Geometry check sheet. Reference: the model listing, model coordinates, mm. Face numbers are marked on the shaded views. Coordinates: 2 decimals unless noted, no trailing zeros. Loops run counter-clockwise (first coordinate to the right, second up) from the corner with the lowest first, then second, coordinate; pieces in that order, holes last. Notation, with made-up numbers: (60, 72.25) -> (116, 72.25) arc R16 ccw to (116, 88.25) -> close; hole circle Ø7 at (-36, -5). An arc over 180 degrees is marked (long way). Answer as a JSON object with one key per item and string values.
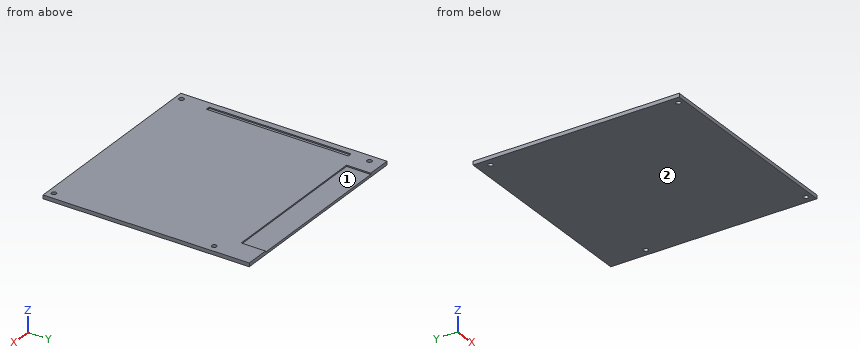
from build123d import *

# Parameters (mm, degrees)
F0_W     = 170
F0_H     = 170
F0_R     = 1.98
F1_DEPTH = 3
F2_W     = 130
F2_H     = 20
F3_DEPTH = 1
F4_W     = 3.516979
F4_H     = 117.000129
F5_DEPTH = 1


with BuildPart() as f1:
    # F0 (on Top) → F1 (new body)
    with BuildSketch(Plane.XY):
        Rectangle(F0_W, F0_H)
        with Locations((-78.65, -80.1)):
            Circle(F0_R, mode=Mode.SUBTRACT)
        with Locations((78.83, -80.1)):
            Circle(F0_R, mode=Mode.SUBTRACT)
        with Locations((-78.65, 74.84)):
            Circle(F0_R, mode=Mode.SUBTRACT)
        with Locations((78.83, 51.98)):
            Circle(F0_R, mode=Mode.SUBTRACT)
    extrude(amount=F1_DEPTH)

    # F2 (on face) → F3 (cut)
    with BuildSketch(Plane.XY.offset(3)):
        with Locations((0, 75)):
            Rectangle(F2_W, F2_H)
    extrude(amount=-F3_DEPTH, mode=Mode.SUBTRACT)

    # F4 (on face) → F5 (cut, through all)
    with BuildSketch(Plane.XY.offset(3)):
        with Locations((-78.040425, 0.470964)):
            Rectangle(F4_W, F4_H)
    extrude(amount=-F5_DEPTH, mode=Mode.SUBTRACT)


solid = f1.part
1. Depth check by flat-ended pin: P1, Ø4, axis at x = -79, y = 6.5, coming from the +Z side; P2, Ø0.5, axis at x = 18, z = 2.5, coming from the +Y side. Enter the tip coordinate at first touch or a pass-through.
Evaluation:
{"P1": "stops at z = 3", "P2": "stops at y = 65"}
2. Section check A-A, the plane y = -80.1. Record the boundary of the cut face in (x, z).
Evaluation:
{"outline": "(-85, 0) -> (-80.63, 0) -> (-80.63, 3) -> (-85, 3) -> close; (-76.67, 0) -> (76.85, 0) -> (76.85, 3) -> (-76.67, 3) -> close; (80.81, 0) -> (85, 0) -> (85, 3) -> (80.81, 3) -> close"}
3. Thickness scan on probe 1 along Y at (x, z) = (78.83, 1); probe 2 along X at (y, z) = (10, 2.1); probe 3 along Z at (x, y) = (-27, 69). Record the ranges inside material, lowest first. Write a range as from..to.
Evaluation:
{"probe 1": "y = -85..-82.08, -78.12..50, 53.96..85", "probe 2": "x = -85..-79.8, -76.28..85", "probe 3": "z = 0..2"}
4. Section check C-C, the plane y = 51.98. Record the boundary of the cut face in (x, z), then the cut area to 3 significant figures.
Evaluation:
{"outline": "(-85, 0) -> (76.85, 0) -> (76.85, 3) -> (-76.28, 3) -> (-76.28, 2) -> (-79.8, 2) -> (-79.8, 3) -> (-85, 3) -> close; (80.81, 0) -> (85, 0) -> (85, 3) -> (80.81, 3) -> close", "area": "495 mm^2"}
5. Section check B-B, the plane z = 2.55. Record the boundary of the cut face in (x, y), then the cut area to 3 significant figures.
Evaluation:
{"outline": "(-85, -85) -> (85, -85) -> (85, 85) -> (65, 85) -> (65, 65) -> (-65, 65) -> (-65, 85) -> (-85, 85) -> close; hole circle Ø3.96 at (-78.65, -80.1); hole circle Ø3.96 at (-78.65, 74.84); hole (-79.8, -58.03) -> (-76.28, -58.03) -> (-76.28, 58.97) -> (-79.8, 58.97) -> close; hole circle Ø3.96 at (78.83, -80.1); hole circle Ø3.96 at (78.83, 51.98)", "area": "25,800 mm^2"}
6. Mould release check, pull along X, two halves, no side actions. Record for the marked faces 1 and 2: released by +X, released by -X, zero draft, split by the parting line, or undercut.
Evaluation:
{"face 1": "undercut", "face 2": "zero draft"}
7. Section check D-D, the plane x = 78.83. Record the boundary of the cut face in (y, z).
Evaluation:
{"outline": "(-85, 0) -> (-82.08, 0) -> (-82.08, 3) -> (-85, 3) -> close; (-78.12, 0) -> (50, 0) -> (50, 3) -> (-78.12, 3) -> close; (53.96, 0) -> (85, 0) -> (85, 3) -> (53.96, 3) -> close"}
